Work out the finished part from the listing and answer in its coordinate system (mm). Round coordinates to 2 decimals unless told otherwise and drop trailing zeros. Order: outer loops, then holes, each group sorted by start corner. A loop starts at its lowest first (then second) coordinate and runs counter-clockwise, first axis right, second up. Notation, with made-up numbers: (25, -32) - (48, -32) arc R27 ccw to (48, 6) - close; hole circle Ø7 at (36, -25.75). An arc over 180 degrees is marked (long way). Answer in a Markdown table with one row per item.
from build123d import *

# Parameters (mm, degrees)
SKETCH1_R           = 2.1828125
BOSS_EXTRUDE1_DEPTH = 6.35
CHAMFER1_SIZE       = 0.396875


with BuildPart() as part:
    # Sketch1 → Boss-Extrude1 (new body)
    with BuildSketch(Plane(origin=(0, 0, 0), x_dir=(1, 0, 0), z_dir=(0, 1, 0))):
        with BuildLine():
            Line((-3.367596045, 3.367596045), (18.213527304, 24.948719395))
            ThreePointArc((18.213527304, 24.948719395), (36.812246699, 69.85), (18.213527304, 114.751280605))
            Line((18.213527304, 114.751280605), (-3.367596045, 136.332403955))
            ThreePointArc((-3.367596045, 136.332403955), (-3.367596045, 143.067596045), (3.367596045, 143.067596045))
            Line((3.367596045, 143.067596045), (24.948719395, 121.486472696))
            ThreePointArc((24.948719395, 121.486472696), (69.85, 102.887753301), (114.751280605, 121.486472696))
            Line((114.751280605, 121.486472696), (136.332403955, 143.067596045))
            ThreePointArc((136.332403955, 143.067596045), (143.067596045, 143.067596045), (143.067596045, 136.332403955))
            Line((143.067596045, 136.332403955), (121.486472696, 114.751280605))
            ThreePointArc((121.486472696, 114.751280605), (102.887753301, 69.85), (121.486472696, 24.948719395))
            Line((121.486472696, 24.948719395), (143.067596045, 3.367596045))
            ThreePointArc((143.067596045, 3.367596045), (143.067596045, -3.367596045), (136.332403955, -3.367596045))
            Line((136.332403955, -3.367596045), (114.751280605, 18.213527304))
            ThreePointArc((114.751280605, 18.213527304), (69.85, 36.812246699), (24.948719395, 18.213527304))
            Line((24.948719395, 18.213527304), (3.367596045, -3.367596045))
            ThreePointArc((3.367596045, -3.367596045), (-3.367596045, -3.367596045), (-3.367596045, 3.367596045))
        make_face()
        with Locations((0, 139.7)):
            Circle(SKETCH1_R, mode=Mode.SUBTRACT)
        Circle(SKETCH1_R, mode=Mode.SUBTRACT)
        with Locations((139.7, 0)):
            Circle(SKETCH1_R, mode=Mode.SUBTRACT)
        with Locations((139.7, 139.7)):
            Circle(SKETCH1_R, mode=Mode.SUBTRACT)
        with BuildLine():
            Line((45.359313119, 52.094505209), (62.665795103, 69.400987194))
            ThreePointArc((62.665795103, 69.400987194), (62.851782297, 69.85), (62.665795103, 70.299012806))
            Line((62.665795103, 70.299012806), (45.359313119, 87.605494791))
            ThreePointArc((45.359313119, 87.605494791), (44.599596932, 87.71027654), (44.293075712, 87.007288174))
            ThreePointArc((44.293075712, 87.007288174), (46.337246699, 69.85), (44.293075712, 52.692711826))
            ThreePointArc((44.293075712, 52.692711826), (44.599596932, 51.98972346), (45.359313119, 52.094505209))
        make_face(mode=Mode.SUBTRACT)
        with BuildLine():
            Line((94.340686881, 87.605494791), (77.034204897, 70.299012806))
            ThreePointArc((77.034204897, 70.299012806), (76.848217703, 69.85), (77.034204897, 69.400987194))
            Line((77.034204897, 69.400987194), (94.340686881, 52.094505209))
            ThreePointArc((94.340686881, 52.094505209), (95.100403068, 51.98972346), (95.406924288, 52.692711826))
            ThreePointArc((95.406924288, 52.692711826), (93.362753301, 69.85), (95.406924288, 87.007288174))
            ThreePointArc((95.406924288, 87.007288174), (95.100403068, 87.71027654), (94.340686881, 87.605494791))
        make_face(mode=Mode.SUBTRACT)
        with BuildLine():
            Line((87.605494791, 45.359313119), (70.299012806, 62.665795103))
            ThreePointArc((70.299012806, 62.665795103), (69.85, 62.851782297), (69.400987194, 62.665795103))
            Line((69.400987194, 62.665795103), (52.094505209, 45.359313119))
            ThreePointArc((52.094505209, 45.359313119), (51.98972346, 44.599596932), (52.692711826, 44.293075712))
            ThreePointArc((52.692711826, 44.293075712), (69.85, 46.337246699), (87.007288174, 44.293075712))
            ThreePointArc((87.007288174, 44.293075712), (87.71027654, 44.599596932), (87.605494791, 45.359313119))
        make_face(mode=Mode.SUBTRACT)
        with BuildLine():
            Line((52.094505209, 94.340686881), (69.400987194, 77.034204897))
            ThreePointArc((69.400987194, 77.034204897), (69.85, 76.848217703), (70.299012806, 77.034204897))
            Line((70.299012806, 77.034204897), (87.605494791, 94.340686881))
            ThreePointArc((87.605494791, 94.340686881), (87.71027654, 95.100403068), (87.007288174, 95.406924288))
            ThreePointArc((87.007288174, 95.406924288), (69.85, 93.362753301), (52.692711826, 95.406924288))
            ThreePointArc((52.692711826, 95.406924288), (51.98972346, 95.100403068), (52.094505209, 94.340686881))
        make_face(mode=Mode.SUBTRACT)
    extrude(amount=BOSS_EXTRUDE1_DEPTH)

    # Chamfer1
    chamfer1_edges = [part.edges().sort_by_distance(p)[0] for p in [
        (125.54184228, 6.35, -132.277034371),
        (69.85, 6.35, -102.887753301),
        (14.15815772, 6.35, -132.277034371),
        (-3.367596045, 6.35, -143.067596045),
        (7.422965629, 6.35, -125.54184228),
        (36.812246699, 6.35, -69.85),
        (7.422965629, 6.35, -14.15815772),
        (-3.367596045, 6.35, 3.367596045),
        (44.599596932, 6.35, -51.98972346),
        (85.687445889, 6.35, -60.747746202),
        (76.848217703, 6.35, -69.85),
        (85.687445889, 6.35, -78.952253798),
        (95.100403068, 6.35, -87.71027654),
        (93.362753301, 6.35, -69.85),
        (95.100403068, 6.35, -51.98972346),
        (78.952253798, 6.35, -85.687445889),
        (69.85, 6.35, -76.848217703),
        (60.747746202, 6.35, -85.687445889),
        (51.98972346, 6.35, -95.100403068),
        (46.337246699, 6.35, -69.85),
        (69.85, 6.35, -93.362753301),
        (87.71027654, 6.35, -95.100403068),
        (69.85, 6.35, -46.337246699),
        (51.98972346, 6.35, -44.599596932),
        (60.747746202, 6.35, -54.012554111),
        (69.85, 6.35, -62.851782297),
        (78.952253798, 6.35, -54.012554111),
        (87.71027654, 6.35, -44.599596932),
        (44.599596932, 6.35, -87.71027654),
        (54.012554111, 6.35, -78.952253798),
        (62.851782297, 6.35, -69.85),
        (54.012554111, 6.35, -60.747746202),
        (-2.1828125, 6.35, -139.7),
        (87.71027654, 0, -44.599596932),
        (-2.1828125, 6.35, 0),
        (78.952253798, 0, -54.012554111),
        (69.85, 0, -62.851782297),
        (60.747746202, 0, -54.012554111),
        (51.98972346, 0, -44.599596932),
        (69.85, 0, -46.337246699),
        (87.71027654, 0, -95.100403068),
        (69.85, 0, -93.362753301),
        (51.98972346, 0, -95.100403068),
        (60.747746202, 0, -85.687445889),
        (69.85, 0, -76.848217703),
        (137.5171875, 6.35, 0),
        (78.952253798, 0, -85.687445889),
        (95.100403068, 0, -51.98972346),
        (93.362753301, 0, -69.85),
        (95.100403068, 0, -87.71027654),
        (85.687445889, 0, -78.952253798),
        (76.848217703, 0, -69.85),
        (85.687445889, 0, -60.747746202),
        (-3.367596045, 0, 3.367596045),
        (7.422965629, 0, -14.15815772),
        (36.812246699, 0, -69.85),
        (137.5171875, 6.35, -139.7),
        (7.422965629, 0, -125.54184228),
        (-3.367596045, 0, -143.067596045),
        (14.15815772, 0, -132.277034371),
        (69.85, 0, -102.887753301),
        (125.54184228, 0, -132.277034371),
        (143.067596045, 0, -143.067596045),
        (132.277034371, 0, -125.54184228),
        (102.887753301, 0, -69.85),
        (132.277034371, 0, -14.15815772),
        (143.067596045, 0, 3.367596045),
        (14.15815772, 6.35, -7.422965629),
        (125.54184228, 0, -7.422965629),
        (69.85, 0, -36.812246699),
        (14.15815772, 0, -7.422965629),
        (137.5171875, 0, -139.7),
        (137.5171875, 0, 0),
        (-2.1828125, 0, 0),
        (-2.1828125, 0, -139.7),
        (54.012554111, 0, -60.747746202),
        (62.851782297, 0, -69.85),
        (54.012554111, 0, -78.952253798),
        (69.85, 6.35, -36.812246699),
        (44.599596932, 0, -87.71027654),
        (46.337246699, 0, -69.85),
        (44.599596932, 0, -51.98972346),
        (125.54184228, 6.35, -7.422965629),
        (143.067596045, 6.35, 3.367596045),
        (132.277034371, 6.35, -14.15815772),
        (102.887753301, 6.35, -69.85),
        (132.277034371, 6.35, -125.54184228),
        (143.067596045, 6.35, -143.067596045),
    ]]
    chamfer(chamfer1_edges, length=CHAMFER1_SIZE)


solid = part.part
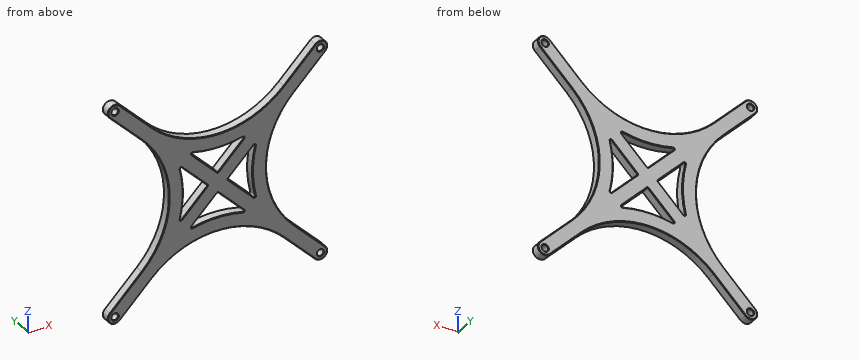
1) Find section C-C, the plane z = -139.7. Give the number of separate pieces and of enclosed holes in the cut face, then the cut area to 3 significant figures.
Filled in:
| item | result |
|---|---|
| separate pieces | 4 |
| enclosed holes | 0 |
| area | 89.2 mm^2 |
2) Find section B-B, the plane z = -6. Give the vertices of the cut face in (x, y).
Filled in:
| item | result |
|---|---|
| outline | (-0.74, 0.4) - (-0.17, 0) - (12.17, 0) - (12.74, 0.4) - (12.74, 5.95) - (12.17, 6.35) - (-0.17, 6.35) - (-0.74, 5.95) - close; (126.96, 0.4) - (127.53, 0) - (139.87, 0) - (140.44, 0.4) - (140.44, 5.95) - (139.87, 6.35) - (127.53, 6.35) - (126.96, 5.95) - close |
3) Find section A-A, the plane x = 15.5. Give the vertices of the cut face in (y, z), then the cut area to 3 significant figures.
Filled in:
| item | result |
|---|---|
| outline | (0, -130.37) - (0.4, -130.94) - (5.95, -130.94) - (6.35, -130.37) - (6.35, -118.03) - (5.95, -117.46) - (0.4, -117.46) - (0, -118.03) - close; (0, -21.67) - (0.4, -22.24) - (5.95, -22.24) - (6.35, -21.67) - (6.35, -9.33) - (5.95, -8.76) - (0.4, -8.76) - (0, -9.33) - close |
| area | 170 mm^2 |
4) Find the intervals of material crossed by probe 1 along Z at (x, y) = (139.7, 3.7); probe 2 along X at (y, z) = (5.5, -78); probe 3 along X at (y, z) = (4.45, 0), in increasing order. Write a range as from..to.
Filled in:
| item | result |
|---|---|
| probe 1 | z = -144.46..-141.88, -137.52..-132.96, -6.74..-2.18, 2.18..4.76 |
| probe 2 | x = 36.29..45.88, 54.96..68.44, 71.26..84.74, 93.82..103.41 |
| probe 3 | x = -4.76..-2.18, 2.18..6.74, 132.96..137.52, 141.88..144.46 |
5) Each of these flat-tipped pins is pushed along its axis until it touches: pin 1 (1 mm diameter, centred on y = 4, z = -82, fed in from +X); pin 2 (5 mm diameter, centred on x = 139.7, z = -139.7, fed in from -Y); pin 3 (3 mm diameter, centred on y = 4.5, z = -120.5, fed in from -X). Where does it stop, or does it pass through?
Filled in:
| item | result |
|---|---|
| pin 1 | stops at x = 104.16 |
| pin 2 | stops at y = 0.08 |
| pin 3 | stops at x = 10.96 |
